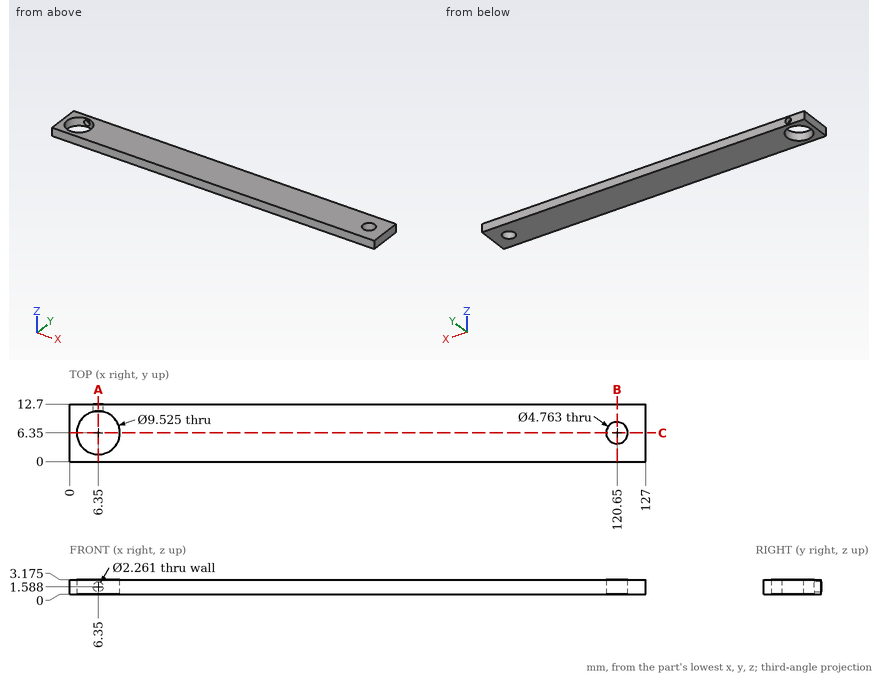
Input: dimensioned drawing with shaded views. Units: mm. Origin: part minimum x, y, z. Round coordinates to 2 decimals unless told otherwise and drop trailing zeros. Order: outer loops, then holes, each group sorted by start corner. A loop starts at its lowest first (then second) coordinate and runs counter-clockwise, first axis right, second up. Notation, with made-up numbers: M 46,17.25 L 76,17.25 A9 ccw 76,33.25 Z; hole C -25.5,8 d6. An arc over 180 degrees is marked long. Use one line per item in the form item = value. Start each with the question number.
Q1. Cut plane A-A (x = 6.35). Return loops of the section in (y, z) (1 decimal).
Q2. Cut plane C-C (y = 6.35). Return loops of the section in (x, z) (1 decimal).
Q3. Cut plane B-B (x = 120.65). Return loops of the section in (y, z) (1 decimal).
Q4. Material intervals for line 1 (Z direction, x = 6.35, y = 11.6) (1 decimal); line 2 (Y direction, x = 120.65, z = 1); line 3 (X direction, y = 3.75, z = 1.55), sorted ascending. Write a range as [from, to].
Geometry results:
q1.outline = M 0,0 L 1.6,0 L 1.6,3.2 L 0,3.2 Z; M 11.1,0 L 12.7,0 L 12.7,0.5 L 11.1,0.5 Z; M 11.1,2.7 L 12.7,2.7 L 12.7,3.2 L 11.1,3.2 Z
q2.outline = M 0,0 L 1.6,0 L 1.6,3.2 L 0,3.2 Z; M 11.1,0 L 118.3,0 L 118.3,3.2 L 11.1,3.2 Z; M 123,0 L 127,0 L 127,3.2 L 123,3.2 Z
q3.outline = M 0,0 L 4,0 L 4,3.2 L 0,3.2 Z; M 8.7,0 L 12.7,0 L 12.7,3.2 L 8.7,3.2 Z
q4.line_1 = [0, 0.5], [2.7, 3.2]
q4.line_2 = [0, 3.97], [8.73, 12.7]
q4.line_3 = [0, 2.36], [10.34, 127]
